```python
from build123d import *

# Parameters (mm, degrees)
F1_DEPTH = 406.4
F2_SIZE  = 22.352
F3_R     = 2.4638
F4_DEPTH = 25.4
F5_R     = 3.2639
F6_DEPTH = 25.4


with BuildPart() as f1:
    # F0 (on Top) → F1 (new body)
    with BuildSketch(Plane.XY):
        with BuildLine():
            ThreePointArc((0, 7.0612), (2.068178, 2.068178), (7.0612, 0))
            Line((7.0612, 0), (31.75, 0))
            Line((31.75, 0), (31.75, 4.7752))
            Line((31.75, 4.7752), (7.0612, 4.7752))
            ThreePointArc((7.0612, 4.7752), (5.444754, 5.444754), (4.7752, 7.0612))
            Line((4.7752, 7.0612), (4.7752, 31.75))
            Line((4.7752, 31.75), (0, 31.75))
            Line((0, 31.75), (0, 7.0612))
        make_face()
    extrude(amount=-F1_DEPTH)

    # F2
    f2_edges = [f1.edges().sort_by_distance(p)[0] for p in [
        (31.75, 2.3876, 0),
        (31.75, 2.3876, -406.4),
    ]]
    chamfer(f2_edges, length=F2_SIZE)

    # F3 (on face) → F4 (cut)
    with BuildSketch(Plane.YZ.offset(4.7752)):
        with Locations((19.4056, -330.2)):
            Circle(F3_R)
        with Locations((19.4056, -76.2)):
            Circle(F3_R)
        with Locations((19.4056, -25.4)):
            Circle(F3_R)
        with Locations((19.4056, -381)):
            Circle(F3_R)
        with Locations((19.4056, -279.4)):
            Circle(F3_R)
        with Locations((19.4056, -228.6)):
            Circle(F3_R)
        with Locations((19.4056, -177.8)):
            Circle(F3_R)
        with Locations((19.4056, -127)):
            Circle(F3_R)
    extrude(amount=-F4_DEPTH, mode=Mode.SUBTRACT)

    # F5 (on face) → F6 (cut)
    with BuildSketch(Plane.XZ):
        with Locations((19.4056, -177.8)):
            Circle(F5_R)
        with Locations((19.4056, -133.35)):
            Circle(F5_R)
        with Locations((19.4056, -88.9)):
            Circle(F5_R)
        with Locations((19.4056, -44.45)):
            Circle(F5_R)
        with Locations((19.4056, -361.95)):
            Circle(F5_R)
        with Locations((19.4056, -317.5)):
            Circle(F5_R)
        with Locations((19.4056, -273.05)):
            Circle(F5_R)
        with Locations((19.4056, -228.6)):
            Circle(F5_R)
    extrude(amount=-F6_DEPTH, mode=Mode.SUBTRACT)


solid = f1.part
```
Check sheet for the modelled part. Datum: model origin and axes. Units: mm. A direction names the side the tool comes from. Give positions to 0.01 mm unless a question says otherwise; leave off trailing zeros. Write each loop counter-clockwise with the first axis right and the second up, starting at its lowest first coordinate (ties: lowest second). Pieces come first, ordered by that corner, then holes. Notation, with made-up numbers: (-34.75, -33) - (-26.75, -33) arc R20 cw to (-26.75, -24) - close; hole circle Ø8 at (-24, 4). An arc over 180 degrees is marked (long way). Answer as a JSON object with one key per item and string values. Group by question number.
1) Sectioned sample at C-C (x = 26). Record the cut outline in (y, z).
2) Sectioned sample at B-B (y = 12). Record the cut outline in (x, z).
3) Depth check by flat-ended pin: P1, Ø7.5, axis at x = 13.5, z = -271.5, coming from the +Y side; P2, Ø8.5, axis at x = 19.41, z = -361.95, coming from the -Y side; P3, Ø5.5, axis at y = 19.41, z = -25.4, coming from the +X side. Enter the tip coordinate at first touch or a pass-through.
4) Access from +Z, -Z, +X, -X, +Y, -Y to the whole of each face (thin tool, end or side, straight path). Record for faces 5 (the face through (18.981, 2.354, -314.264)), 6 (the face through (4.775, 19, -200)).
5) Sectioned sample at A-A (z = -113.5). Record the cut outline in (x, y), then the cut area to 3 significant figures.
6) Release check for a two-part mould opening along X. For faces 1 (the face through (19, 0, -200)), 2 (the face through (18.981, 2.354, -174.564)), 3 (the face through (2.014, 2.123, -200.355)), 4 (the face through (18.698, 2.354, -276.236)) record: pulls with the +X half, pulls with the -X half, needs draft (parallel to the pull), parting line crosses it, or undercut.
7) Thickness scan on probe 1 along Y at (x, z) = (30, -24); probe 2 along Y at (x, z) = (1, -279). Record the ranges inside material, lowest first. Write a range as from..to.
Geometry results:
{
 "1": {"outline": "(0, -389.8) - (4.78, -389.8) - (4.78, -16.6) - (0, -16.6) - close"},
 "2": {"outline": "(0, -406.4) - (4.78, -406.4) - (4.78, 0) - (0, 0) - close"},
 "3": {"P1": "stops at y = 4.78", "P2": "stops at y = 0", "P3": "stops at x = 4.78"},
 "4": {"face 5": "+Y, -Y", "face 6": "+Z, -Z, +X, +Y"},
 "5": {"outline": "(0, 7.06) arc R7.06 ccw to (7.06, 0) - (31.75, 0) - (31.75, 4.78) - (7.06, 4.78) arc R2.29 cw to (4.78, 7.06) - (4.78, 31.75) - (0, 31.75) - close", "area": "271 mm^2"},
 "6": {"face 1": "needs draft", "face 2": "undercut", "face 3": "pulls with the -X half", "face 4": "undercut"},
 "7": {"probe 1": "y = 0..4.78", "probe 2": "y = 3.44..16.97, 21.84..31.75"}
}
